from build123d import *

# Parameters (mm, degrees)
SKETCH1_W           = 63.5
SKETCH1_H           = 28.7782
BOSS_EXTRUDE1_DEPTH = 7.62
FILLET1_R           = 2.54
BOSS_EXTRUDE2_START = 31.75
SKETCH2_R           = 1.651
BOSS_EXTRUDE2_DEPTH = 6.35
BOSS_EXTRUDE3_START = -31.75
SKETCH2_2_R         = 1.651
BOSS_EXTRUDE3_DEPTH = 6.35


with BuildPart() as part:
    # Sketch1 → Boss-Extrude1 (new body, symmetric)
    with BuildSketch(Plane(origin=(0, 0, 0), x_dir=(1, 0, 0), z_dir=(0, 1, 0))):
        Rectangle(SKETCH1_W, SKETCH1_H)
    extrude(amount=BOSS_EXTRUDE1_DEPTH, both=True)

    # Fillet1
    fillet1_edges = [part.edges().sort_by_distance(p)[0] for p in [
        (-31.75, 7.62, 0),
        (0, 7.62, 14.3891),
        (31.75, 7.62, 0),
        (0, -7.62, 14.3891),
        (-31.75, -7.62, 0),
        (0, -7.62, -14.3891),
        (31.75, -7.62, 0),
        (31.75, 0, 14.3891),
        (-31.75, 0, 14.3891),
        (-31.75, 0, -14.3891),
        (31.75, 0, -14.3891),
        (0, 7.62, -14.3891),
    ]]
    fillet(fillet1_edges, radius=FILLET1_R)

    # Sketch2 → Boss-Extrude2 (add)
    with BuildSketch(Plane(origin=(0, 0, 0), x_dir=(0, 0, -1), z_dir=(1, 0, 0)).offset(BOSS_EXTRUDE2_START)):
        Circle(SKETCH2_R)
        with Locations((10.16, 0)):
            Circle(SKETCH2_R)
        with Locations((-10.16, 0)):
            Circle(SKETCH2_R)
    extrude(amount=BOSS_EXTRUDE2_DEPTH)

    # Sketch2<2> → Boss-Extrude3 (add)
    with BuildSketch(Plane(origin=(0, 0, 0), x_dir=(0, 0, -1), z_dir=(1, 0, 0)).offset(BOSS_EXTRUDE3_START)):
        with Locations((10.16, 0)):
            Circle(SKETCH2_2_R)
        with Locations((-10.16, 0)):
            Circle(SKETCH2_2_R)
    extrude(amount=-BOSS_EXTRUDE3_DEPTH)


solid = part.part
The model under review builds one solid part; all positions refer to its coordinate system, in mm. A direction names the side the tool comes from. Round coordinates to 2 decimals unless told otherwise and drop trailing zeros. Order: outer loops, then holes, each group sorted by start corner. A loop starts at its lowest first (then second) coordinate and runs counter-clockwise, first axis right, second up. Notation, with made-up numbers: (12.25, 58.5) -> (34.25, 58.5) arc R30 cw to (34.25, 92.5) -> close; hole circle Ø7 at (-31, -31.5). An arc over 180 degrees is marked (long way). Return JSON: item names as keys, results as strings.
1. Take a section at B-B (y = -4). Write out the cut boundary in (x, z).
Answer block:
{"outline": "(-31.75, -11.85) arc R2.54 ccw to (-29.21, -14.39) -> (29.21, -14.39) arc R2.54 ccw to (31.75, -11.85) -> (31.75, 11.85) arc R2.54 ccw to (29.21, 14.39) -> (-29.21, 14.39) arc R2.54 ccw to (-31.75, 11.85) -> close"}
2. For faces 1 (the face through (-31.026, -0.071, -13.625)), 2 (the face through (34.88, 0.07, -8.51)), list the 3-axis set-ups (+Z, -Z, +X, -X, +Y, -Y) from which the entire face can be reached by the end or side of a thin tool; tool diameter is ignored.
Answer block:
{"face 1": "-Z, -X, +Y, -Y", "face 2": "+X"}
3. For L1, parallel to Y at x = -29.5, z = -3; L2, parallel to X at y = 3.5, z = -3; L3, parallel to Y at x = 7, z = 12.75, list the stretches that pass through material, from the lowest coordinate up. Write a range as [from, to].
Answer block:
{"L1": "y = [-7.6, 7.6]", "L2": "x = [-31.75, 31.75]", "L3": "y = [-7.45, 7.45]"}
4. The part is to be moulded in two halves that separate along Z. For faces 3 (the face through (-34.88, 0.07, 11.81)), 4 (the face through (38.1, 0, 0)), 5 (the face through (0.409, 6.896, -13.625)), 6 (the face through (-34.88, 0.07, -8.51)), say which applies: +Z half, -Z half, draft (parallel to the pull), parting line (faces both ways), or undercut.
Answer block:
{"face 3": "undercut", "face 4": "draft", "face 5": "-Z half", "face 6": "undercut"}
5. Insertion check: P1, Ø6, axis at y = -6, z = 1.5, coming from the +X side; P2, Ø3, axis at y = 2.5, z = 5, coming from the -X side. Each pin has a flat end and moves straight along its axis. Give the tip position at first contact, or say it passes through.
Answer block:
{"P1": "stops at x = 31.75", "P2": "stops at x = -31.75"}
6. Take a section at A-A (z = 0). Write out the cut boundary in (x, y), then the cut area to 3 significant figures.
Answer block:
{"outline": "(-31.75, -5.08) arc R2.54 ccw to (-29.21, -7.62) -> (29.21, -7.62) arc R2.54 ccw to (31.75, -5.08) -> (31.75, -1.65) -> (38.1, -1.65) -> (38.1, 1.65) -> (31.75, 1.65) -> (31.75, 5.08) arc R2.54 ccw to (29.21, 7.62) -> (-29.21, 7.62) arc R2.54 ccw to (-31.75, 5.08) -> close", "area": "983 mm²"}
7. Take a section at D-D (z = 10.16). Write out the cut boundary in (x, y), then the cut area to 3 significant figures.
Answer block:
{"outline": "(-38.1, -1.65) -> (-31.75, -1.65) -> (-31.75, -5.08) arc R2.54 ccw to (-29.21, -7.62) -> (29.21, -7.62) arc R2.54 ccw to (31.75, -5.08) -> (31.75, -1.65) -> (38.1, -1.65) -> (38.1, 1.65) -> (31.75, 1.65) -> (31.75, 5.08) arc R2.54 ccw to (29.21, 7.62) -> (-29.21, 7.62) arc R2.54 ccw to (-31.75, 5.08) -> (-31.75, 1.65) -> (-38.1, 1.65) -> close", "area": "1,000 mm²"}
